Work out the finished part from the listing and answer in its coordinate system (mm). Round coordinates to 2 decimals unless told otherwise and drop trailing zeros. Write each loop counter-clockwise with the first axis right and the second up, starting at its lowest first coordinate (ties: lowest second). Pieces come first, ordered by that corner, then holes. Notation, with made-up numbers: (49, 70) -> (78, 70) arc R12 ccw to (78, 89) -> close; hole circle Ø9 at (31, 6.25). An arc over 180 degrees is marked (long way). One line per item, written item: value.
```python
from build123d import *

# Parameters (mm, degrees)
F0_W     = 21.5146457776
F0_H     = 6
F1_DEPTH = 4
F2_W     = 0.5
F2_H     = 4
F2_W_2   = 2
F2_H_2   = 1.25
F3_DEPTH = 0.4


# Not quite as in the source:
# - a feature names something its author has since deleted; it is built from what else it names


with BuildPart() as f1:
    # F0 (on Front) → F1 (new body)
    with BuildSketch(Plane.XZ):
        with BuildLine():
            ThreePointArc((-5, 20), (0, 15), (5, 20))
            Line((5, 20), (-5, 20))
        make_face()
        with BuildLine():
            Line((-5, 20), (5, 20))
            ThreePointArc((5, 20), (4.8783151775, 21.0963763172), (4.5191835885, 22.1393876913))
            ThreePointArc((4.5191835885, 22.1393876913), (0, 25), (-4.5191835885, 22.1393876913))
            ThreePointArc((-4.5191835885, 22.1393876913), (-4.8783151775, 21.0963763172), (-5, 20))
        make_face()
        with BuildLine():
            Line((5.5319726474, 20), (5, 20))
            ThreePointArc((5, 20), (0, 15), (-5, 20))
            Line((-5, 20), (-5.5319726474, 20))
            Line((-5.5319726474, 20), (-15, 0))
            Line((-15, 0), (-10.795, 0))
            Line((-10.795, 0), (-10.795, 3))
            Line((-10.795, 3), (10.795, 3))
            Line((10.795, 3), (10.795, 0))
            Line((10.795, 0), (15, 0))
            Line((15, 0), (5.5319726474, 20))
        make_face()
        with BuildLine():
            Line((15, -16.4057657868), (15, 0))
            Line((15, 0), (10.795, 0))
            Line((10.795, 0), (10.795, -3))
            Line((10.795, -3), (-10.795, -3))
            Line((-10.795, -3), (-10.795, 0))
            Line((-10.795, 0), (-15, 0))
            Line((-15, 0), (-15, -16.4057657868))
            ThreePointArc((-15, -16.4057657868), (-13.5355339059, -19.9412996927), (-10, -21.4057657868))
            Line((-10, -21.4057657868), (10, -21.4057657868))
            ThreePointArc((10, -21.4057657868), (13.5355339059, -19.9412996927), (15, -16.4057657868))
        make_face()
        with Locations((-0.0376771112, -12.0637425241)):
            Rectangle(F0_W, F0_H, mode=Mode.SUBTRACT)
        with BuildLine():
            Line((-5.5319726474, 20), (-5, 20))
            ThreePointArc((-5, 20), (-4.8783151775, 21.0963763172), (-4.5191835885, 22.1393876913))
            Line((-4.5191835885, 22.1393876913), (-5.5319726474, 20))
        make_face()
        with BuildLine():
            ThreePointArc((4.5191835885, 22.1393876913), (4.8783151775, 21.0963763172), (5, 20))
            Line((5, 20), (5.5319726474, 20))
            Line((5.5319726474, 20), (4.5191835885, 22.1393876913))
        make_face()
    extrude(amount=F1_DEPTH)

    # F2 (on face) → F3 (cut)
    with BuildSketch(Plane.XZ.offset(4)):
        Polygon((-10.4092183411, -4.0046597868), (-10.9092183411, -4.0046597868), (-10.9092183411, -8.0046597868), (-10.4092183411, -8.0046597868), (-10.4092183411, -4.5046597868), (-10.3992183411, -4.5046597868), (-9.4092183411, -5.54676505), (-8.4192183411, -4.5046597868), (-8.4092183411, -4.5046597868), (-8.4092183411, -8.0046597868), (-7.9092183411, -8.0046597868), (-7.9092183411, -4.0046597868), (-8.4092183411, -4.0046597868), (-8.6092183411, -4.0046597868), (-9.4092183411, -4.84676505), (-10.2092183411, -4.0046597868), align=None)
        Polygon((-4.2092183411, -5.0046597868), (-7.2092183411, -5.0046597868), (-7.2092183411, -8.0046597868), (-4.2092183411, -8.0046597868), (-4.2092183411, -7.2046597868), (-4.7092183411, -7.2046597868), (-4.7092183411, -7.5046597868), (-6.7092183411, -7.5046597868), (-6.7092183411, -5.5046597868), (-4.7092183411, -5.5046597868), (-4.7092183411, -5.8046597868), (-4.2092183411, -5.8046597868), align=None)
        Polygon((-0.7092183411, -4.0046597868), (-3.7092183411, -4.0046597868), (-3.7092183411, -8.0046597868), (-3.2092183411, -8.0046597868), (-3.2092183411, -6.2546597868), (-1.7092183411, -6.2546597868), (-1.7092183411, -5.7546597868), (-3.2092183411, -5.7546597868), (-3.2092183411, -4.5046597868), (-0.7092183411, -4.5046597868), align=None)
        with Locations((0.0407816589, -6.0046597868)):
            Rectangle(F2_W, F2_H)
        Polygon((3.7907816589, -4.0046597868), (0.7907816589, -4.0046597868), (0.7907816589, -8.0046597868), (1.2907816589, -8.0046597868), (1.2907816589, -6.2546597868), (3.0764354139, -8.0046597868), (3.7907816589, -8.0046597868), (2.0051279039, -6.2546597868), (3.7907816589, -6.2546597868), align=None)
        with Locations((2.2907816589, -5.1296597868)):
            Rectangle(F2_W_2, F2_H_2, mode=Mode.SUBTRACT)
        Polygon((7.2907816589, -4.0046597868), (4.2907816589, -4.0046597868), (4.2907816589, -8.0046597868), (7.2907816589, -8.0046597868), (7.2907816589, -7.5046597868), (4.7907816589, -7.5046597868), (4.7907816589, -6.2546597868), (6.2907816589, -6.2546597868), (6.2907816589, -5.7546597868), (4.7907816589, -5.7546597868), (4.7907816589, -4.5046597868), (7.2907816589, -4.5046597868), align=None)
        Polygon((10.7907816589, -4.0046597868), (7.7907816589, -4.0046597868), (7.7907816589, -6.2546597868), (10.2907816589, -6.2546597868), (10.2907816589, -7.5046597868), (7.7907816589, -7.5046597868), (7.7907816589, -8.0046597868), (10.7907816589, -8.0046597868), (10.7907816589, -5.7546597868), (8.2907816589, -5.7546597868), (8.2907816589, -4.5046597868), (10.7907816589, -4.5046597868), align=None)
    extrude(amount=-F3_DEPTH, mode=Mode.SUBTRACT)


solid = f1.part
```
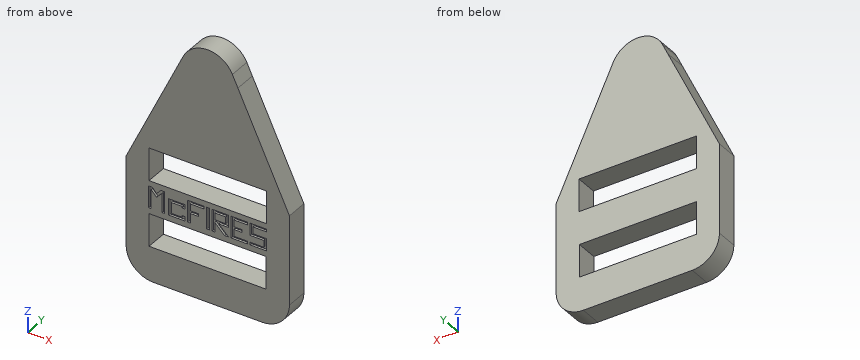
(1) Flat-ended cylindrical pins translate along their axes: pin 1 Ø1.5 at (x, y) = (-6, -3) entering from +Z; pin 2 Ø2 at (y, z) = (-1, 14) entering from -X; pin 3 Ø2 at (x, y) = (-3.5, -3.5) entering from +Z. Find the tip coordinate at first contact, or state that the pin passes through.
Reported:
pin 1: stops at z = 20.6
pin 2: stops at x = -8.85
pin 3: stops at z = 24.33
(2) Find section C-C on x = 11.75. Give the vertices of the cut face in (y, z), plus the area to 3 significant figures.
Reported:
outline: (-4, -21.09) -> (0, -21.09) -> (0, 6.87) -> (-4, 6.87) -> close
area: 112 mm2
(3) Find section B-B on y = -3. Give the vertices of the cut face in (x, z) (3 decimals).
Reported:
outline: (-15, -16.406) arc R5 ccw to (-10, -21.406) -> (10, -21.406) arc R5 ccw to (15, -16.406) -> (15, 0) -> (4.519, 22.139) arc R5 ccw to (-4.519, 22.139) -> (-15, 0) -> close; hole (-10.795, -15.064) -> (10.72, -15.064) -> (10.72, -9.064) -> (-10.795, -9.064) -> close; hole (-10.795, -3) -> (10.795, -3) -> (10.795, 3) -> (-10.795, 3) -> close
(4) Consider probe 1 along X at (y, z) = (-0.4, -9.5) (3 decimals); probe 2 along Z at (x, y) = (9, -0.55); probe 3 along Z at (x, y) = (-4.25, -2.5). Determine where each line is inside the solid, lowest interval first.
Reported:
probe 1: x = -15 to -10.795, 10.72 to 15
probe 2: z = -21.41 to -15.06, -9.06 to -3, 3 to 12.67
probe 3: z = -21.41 to -15.06, -9.06 to -3, 3 to 22.63
(5) Find section A-A on z = -12.5. Give the vertices of the cut face in (x, y) (3 decimals), plus the area to 3 significant figures.
Reported:
outline: (-15, -4) -> (-10.795, -4) -> (-10.795, 0) -> (-15, 0) -> close; (10.72, -4) -> (15, -4) -> (15, 0) -> (10.72, 0) -> close
area: 33.9 mm2
(6) Find section D-D on z = -19. Give the vertices of the cut face in (x, y).
Reported:
outline: (-14.27, -4) -> (14.27, -4) -> (14.27, 0) -> (-14.27, 0) -> close
